For this review, take the finished solid that the model builds, in its own axes (mm). Give positions to 0.01 mm unless a question says otherwise; leave off trailing zeros. Write each loop counter-clockwise with the first axis right and the second up, starting at its lowest first coordinate (ties: lowest second). Pieces come first, ordered by that corner, then holes. Notation, with made-up numbers: M 67.5,-19.75 L 93.5,-19.75 A21 cw 93.5,4.25 Z; hole C -21,83 d11. An arc over 180 degrees is marked long. Answer as a JSON object with one key per item and string values. Group by question number.
```python
from build123d import *

# Parameters (mm, degrees)
SKETCH1_W                        = 228.6
SKETCH1_H                        = 25.4
BOSS_EXTRUDE1_DEPTH              = 9.525
F_8_CLEARANCE_HOLE1_D            = 4.4958
F_8_CLEARANCE_HOLE1_DEPTH        = 25.4
F_8_CLEARANCE_HOLE1_TIP          = 1.350674586
F_8_CLEARANCE_HOLE2_D            = 4.4958
F_8_CLEARANCE_HOLE2_DEPTH        = 19.05
F_8_CLEARANCE_HOLE2_TIP          = 1.350674586
CHAMFER1_SIZE                    = 0.508
F_4_CLEARANCE_HOLE1_D            = 3.2639
F_4_CLEARANCE_HOLE2_D            = 3.2639
F_4_CLEARANCE_HOLE2_DEPTH        = 9.525
F_1_8_0_125_DIAMETER_HOLE1_D     = 3.175
F_1_8_0_125_DIAMETER_HOLE1_DEPTH = 9.525


with BuildPart() as part:
    # Sketch1 → Boss-Extrude1 (new body)
    with BuildSketch(Plane.XY):
        with Locations((-114.3, 12.7)):
            Rectangle(SKETCH1_W, SKETCH1_H)
    extrude(amount=BOSS_EXTRUDE1_DEPTH)

    # #8 Clearance Hole1
    with Locations(Plane.XY.offset(9.525)):
        with Locations((-6.35, 6.35), (-6.35, 19.05)):
            Hole(F_8_CLEARANCE_HOLE1_D / 2, depth=F_8_CLEARANCE_HOLE1_DEPTH)
            with Locations((0, 0, -(F_8_CLEARANCE_HOLE1_DEPTH + F_8_CLEARANCE_HOLE1_TIP / 2))):  # 118° drill point
                Cone(0, F_8_CLEARANCE_HOLE1_D / 2, F_8_CLEARANCE_HOLE1_TIP, mode=Mode.SUBTRACT)

    # #8 Clearance Hole2
    with Locations(Plane.XY.offset(9.525)):
        with Locations((-141.2875, 12.7)):
            Hole(F_8_CLEARANCE_HOLE2_D / 2, depth=F_8_CLEARANCE_HOLE2_DEPTH)
            with Locations((0, 0, -(F_8_CLEARANCE_HOLE2_DEPTH + F_8_CLEARANCE_HOLE2_TIP / 2))):  # 118° drill point
                Cone(0, F_8_CLEARANCE_HOLE2_D / 2, F_8_CLEARANCE_HOLE2_TIP, mode=Mode.SUBTRACT)

    # Chamfer1
    chamfer1_edges = [part.edges().sort_by_distance(p)[0] for p in [
        (-228.6, 12.7, 9.525),
        (0, 12.7, 9.525),
        (-228.6, 12.7, 0),
        (0, 12.7, 0),
        (0, 0, 4.7625),
        (-228.6, 0, 4.7625),
        (-228.6, 25.4, 4.7625),
        (0, 25.4, 4.7625),
    ]]
    chamfer(chamfer1_edges, length=CHAMFER1_SIZE)

    # #4 Clearance Hole1 (through all)
    with Locations(Plane(origin=(0, 0, 0), x_dir=(-1, 0, 0), z_dir=(0, 0, -1))):
        with Locations((96.8375, 12.7), (46.0375, 12.7)):
            Hole(F_4_CLEARANCE_HOLE1_D / 2)

    # #4 Clearance Hole2
    with Locations(Plane.XY.offset(9.525)):
        with Locations((-217.4875, 12.7), (-192.0875, 12.7)):
            Hole(F_4_CLEARANCE_HOLE2_D / 2, depth=F_4_CLEARANCE_HOLE2_DEPTH)

    # 1/8 (0.125) Diameter Hole1
    with Locations(Plane.XY.offset(9.525)):
        with Locations((-19.05, 19.05), (-69.85, 19.05), (-120.65, 6.35)):
            Hole(F_1_8_0_125_DIAMETER_HOLE1_D / 2, depth=F_1_8_0_125_DIAMETER_HOLE1_DEPTH)


solid = part.part
```
Item 1: Consider section A-A (x = -141.5). Give the boundary of the cut face in (y, z) (3 decimals).
Item 2: Consider section B-B (z = 7). State how many separate pieces and enclosed holes the cut face has, plus the area to 3 significant figures.
Item 3: Draft analysis for pull direction Y (two halves, no side actions). For faces 1 (the cylindrical face through (-8.5, 19.7, 4.7)), 2 (the flat face through (-228.6, 13, 5)), 3 (the flat face through (-116, 25.4, 5)), state which applies: released by +Y, released by -Y, zero draft, split by the parting line, or undercut.
Item 4: To check wall thickness, follow probe 1 along Y at (x, z) = (-6.35, 2); probe 2 along Y at (x, z) = (-97, 0.5); probe 3 along X at (y, z) = (5.5, 8). State the ranges of each line that lie inside material, in increasing order.
Result set:
{
 "1": {"outline": "M 0,0 L 10.462,0 L 10.462,9.525 L 0,9.525 Z; M 14.938,0 L 25.4,0 L 25.4,9.525 L 14.938,9.525 Z"},
 "2": {"separate pieces": "1", "enclosed holes": "10", "area": "5,700 mm^2"},
 "3": {"face 1": "undercut", "face 2": "zero draft", "face 3": "released by +Y"},
 "4": {"probe 1": "y = 0 to 4.1, 8.6 to 16.8, 21.3 to 25.4", "probe 2": "y = 0 to 11.08, 14.32 to 25.4", "probe 3": "x = -228.6 to -121.99, -119.31 to -8.43, -4.27 to 0"}
}
